Here's how the part is built. I have some questions about the finished solid (model axes, mm). A direction names the side the tool comes from. Give positions to 0.01 mm unless a question says otherwise; leave off trailing zeros. Loops run counter-clockwise (first coordinate to the right, second up) from the corner with the lowest first, then second, coordinate; pieces in that order, holes last. Notation, with made-up numbers: (30.25, 88.5) - (74.25, 88.5) arc R25 cw to (74.25, 109.5) - close; hole circle Ø7 at (4.25, -20). An arc over 180 degrees is marked (long way). Return JSON: item names as keys, results as strings. Group by question number.
(1) If we section it at C-C (z = 21): Please give me the cut outline in (x, y).
(2) If we section it at A-A (x = 32.5): Please give me the cut outline in (y, z).
(3) I need wall thicknesses on probe 1 along X at (y, z) = (-32, 21.5); probe 2 along Z at (x, y) = (33.5, -13); probe 3 along Y at (x, z) = (5.5, 17). Which ranges of each line are inside material? Lowest first, please. Write a range as [from, to].
(4) For P1, Ø1.5, axis at x = 37, y = -24, coming from the +Z side; P2, Ø5, axis at x = 30.5, z = 39.5, coming from the -Y side; P3, Ø2, axis at x = 21.5, y = -16, coming from the +Z side, each with a flat end and sliding along its axis, tell me the tip position at first contact or that it passes through.
(5) On a 3-axis mill with a long thin cutter (end or side, diameter ignored), from which of +Z, -Z, +X, -X, +Y, -Y can I reach the whole of each face in a straight line? I mean faces 1 (the flat face through (25, -31, 24.13)), 2 (the flat face through (25, 0, 25)), 3 (the flat face through (50.8, -12, 12)), 4 (the flat face through (35.719, -36, 15)), 5 (the flat face through (15.081, -36, 15)). Say none if no direction works.
(6) If we section it at D-D (x = 7): Please give me the cut outline in (y, z).
(7) If we section it at B-B (y = -46): Please give me the cut outline in (x, z), then the cut area to 3 significant figures.
```python
from build123d import *

# Parameters (mm, degrees)
F1_DEPTH = 50.8
F2_DEPTH = 35.71875
F3_DEPTH = 15.08125


with BuildPart() as f1:
    # F0 (on Right) → F1 (new body)
    with BuildSketch(Plane.YZ):
        with BuildLine():
            Line((-50.8, 0), (0, 0))
            Line((0, 0), (0, 24.13))
            Line((0, 24.13), (-11.7745487484, 24.13))
            ThreePointArc((-11.7745487484, 24.13), (-29.0316591308, 8.4169932564), (-50.8, 0))
        make_face()
        with BuildLine():
            Line((-11.7745487484, 24.13), (0, 24.13))
            Line((0, 24.13), (0, 50.8))
            ThreePointArc((0, 50.8), (-4.3360005943, 36.7801275312), (-11.7745487484, 24.13))
        make_face()
    extrude(amount=F1_DEPTH)

    # F0 (on Right) → F2 (join)
    with BuildSketch(Plane.YZ):
        with BuildLine():
            Line((-11.7745487484, 24.13), (0, 24.13))
            Line((0, 24.13), (0, 50.8))
            ThreePointArc((0, 50.8), (-4.3360005943, 36.7801275312), (-11.7745487484, 24.13))
        make_face()
        with BuildLine():
            Line((-50.8, 24.13), (-50.8, 0))
            ThreePointArc((-50.8, 0), (-29.0316591308, 8.4169932564), (-11.7745487484, 24.13))
            Line((-11.7745487484, 24.13), (-50.8, 24.13))
        make_face()
        with BuildLine():
            Line((-50.8, 0), (0, 0))
            Line((0, 0), (0, 24.13))
            Line((0, 24.13), (-11.7745487484, 24.13))
            ThreePointArc((-11.7745487484, 24.13), (-29.0316591308, 8.4169932564), (-50.8, 0))
        make_face()
    extrude(amount=F2_DEPTH)

    # F0 (on Right) → F3 (cut)
    with BuildSketch(Plane.YZ):
        with BuildLine():
            Line((-50.8, 24.13), (-50.8, 0))
            ThreePointArc((-50.8, 0), (-29.0316591308, 8.4169932564), (-11.7745487484, 24.13))
            Line((-11.7745487484, 24.13), (-50.8, 24.13))
        make_face()
    extrude(amount=F3_DEPTH, mode=Mode.SUBTRACT)


solid = f1.part
```
Values:
{
 "1": {"outline": "(0, -14.3) - (15.08, -14.3) - (15.08, -50.8) - (35.72, -50.8) - (35.72, -14.3) - (50.8, -14.3) - (50.8, 0) - (0, 0) - close"},
 "2": {"outline": "(-50.8, 0) - (0, 0) - (0, 50.8) arc R63.5 cw to (-11.77, 24.13) - (-50.8, 24.13) - close"},
 "3": {"probe 1": "[15.08, 35.72]", "probe 2": "[0, 24.13]", "probe 3": "[-18.06, 0]"},
 "4": {"P1": "z = 12.45", "P2": "y = -4.24", "P3": "z = 24.13"},
 "5": {"face 1": "+Z, +X, -X, -Y", "face 2": "+Z, -Z, +X, -X, +Y", "face 3": "+Z, -Z, +X, +Y, -Y", "face 4": "+Z, +X, -Y", "face 5": "+Z, -X, -Y"},
 "6": {"outline": "(-50.8, 0) - (0, 0) - (0, 50.8) arc R63.5 cw to start"},
 "7": {"outline": "(0, 0) - (50.8, 0) - (50.8, 1.09) - (35.72, 1.09) - (35.72, 24.13) - (15.08, 24.13) - (15.08, 1.09) - (0, 1.09) - close", "area": "531 mm2"}
}
